```python
from build123d import *

# Parameters (mm, degrees)
ESQUISSE1_W             = 40
ESQUISSE1_H             = 35
BOSS_EXTRU_1_DEPTH      = 4
ESQUISSE2_R             = 10
ENL_V_MAT_EXTRU_1_DEPTH = 2
ENL_V_MAT_EXTRU_2_DEPTH = 27.874709301
BOSS_EXTRU_2_DEPTH      = 100
BOSS_EXTRU_2_DEPTH_BACK = 9
ESQUISSE4_R             = 7
ESQUISSE5_R             = 6
ENL_V_MAT_EXTRU_5_DEPTH = 99
ENL_V_MAT_EXTRU_9_DEPTH = 99


with BuildPart() as part:
    # Esquisse1 → Boss.-Extru.1 (new body)
    with BuildSketch(Plane(origin=(0, 0, 0), x_dir=(0, 0, -1), z_dir=(1, 0, 0))):
        Rectangle(ESQUISSE1_W, ESQUISSE1_H)
    extrude(amount=BOSS_EXTRU_1_DEPTH)

    # Esquisse2 → Enlèv. mat.-Extru.1 (cut)
    with BuildSketch(Plane.ZY):
        Circle(ESQUISSE2_R)
    extrude(amount=-ENL_V_MAT_EXTRU_1_DEPTH, mode=Mode.SUBTRACT)

    # Esquisse3 → Enlèv. mat.-Extru.2 (cut, through all)
    with BuildSketch(Plane.ZY):
        with BuildLine():
            Line((0, -17.5), (20, -17.5))
            Line((20, -17.5), (20, 17.5))
            Line((20, 17.5), (0, 17.5))
            ThreePointArc((0, 17.5), (17.5, 0), (0, -17.5))
        make_face()
    extrude(amount=-ENL_V_MAT_EXTRU_2_DEPTH, mode=Mode.SUBTRACT)

    # Esquisse4 → Boss.-Extru.2 (add, two sides: drawn at the far end of the back side and taken through both)
    with BuildSketch(Plane(origin=(0, 0, -20), x_dir=(-1, 0, 0), z_dir=(0, 0, -1)).offset(-BOSS_EXTRU_2_DEPTH_BACK)):
        with Locations((-6, 0)):
            Circle(ESQUISSE4_R)
    extrude(amount=BOSS_EXTRU_2_DEPTH + BOSS_EXTRU_2_DEPTH_BACK)

    # Esquisse5 → Enlèv. mat.-Extru.5 (cut)
    with BuildSketch(Plane(origin=(0, 0, -120), x_dir=(-1, 0, 0), z_dir=(0, 0, -1))):
        with Locations((-6, 0)):
            Circle(ESQUISSE5_R)
    extrude(amount=-ENL_V_MAT_EXTRU_5_DEPTH, mode=Mode.SUBTRACT)

    # Esquisse10 → Enlèv. mat.-Extru.9 (cut)
    with BuildSketch(Plane.XY.offset(-11)):
        with BuildLine():
            Line((6, -4), (6, 4))
            ThreePointArc((6, 4), (10, 0), (6, -4))
        make_face()
    extrude(amount=-ENL_V_MAT_EXTRU_9_DEPTH, mode=Mode.SUBTRACT)


solid = part.part
```
Read the model definition and answer for the solid it produces. Units are mm, in the model's axes. A direction names the side the tool comes from. Give positions to 0.01 mm unless a question says otherwise; leave off trailing zeros. Order: outer loops, then holes, each group sorted by start corner. A loop starts at its lowest first (then second) coordinate and runs counter-clockwise, first axis right, second up.
(1) Straight lines are drawn through the part: L1, parallel to Y at x = 6, z = -72.5; L2, parallel to X at y = -5, z = -96; L3, parallel to X at y = -2.5, z = -35.5. For each, find the intervals that lie inside material, in ascending order.
(2) For a pull along X with two mould halves and no side action, classify faces 6 (the flat face through (2, 0, 0)), 7 (the flat face through (5, 0, -21)), 8 (the cylindrical face through (1.972, 0.385, 17.496)) as released by +X, released by -X, zero draft, split by the parting line, or undercut.
(3) Find section D-D (y = -8.5). Give the vertices of the cut face in (x, z).
(4) Find section B-B (x = 7.5). Give the vertices of the cut face in (y, z).
(5) Find section C-C (z = -37.5). Give the vertices of the cut face in (x, y).
(6) Find section A-A (y = 0). Give the vertices of the cut face in (x, z).
(7) For faces 1 (the cylindrical face through (0.99, -9.76, -2.17)), 2 (the flat face through (5.6, 0.1, -11)), 3 (the flat face through (2, -17.5, -10)), 4 (the flat face through (6, 0, -16)), 5 (the cylindrical face through (13, 0, -65)), determine the directions among +Z, -Z, +X, -X, +Y, -Y from which every point of the face is accessible in a straight line to the end or side of a thin tool.
(8) Given pin 1 (1 mm diameter, centred on x = 1, y = -10.5, fed in from +Z); pin 2 (1.2 mm diameter, centred on x = 1, y = 12.5, fed in from -Z); pin 3 (2 mm diameter, centred on y = 6, z = -63.5, fed in from +X), each flat-ended and moving along its own axis, determine where each tip first touches the part or whether it passes through.
Result sheet:
1. L1: y = -7 to -6, 6 to 7
1. L2: x = 1.1 to 2.68, 9.32 to 10.9
1. L3: x = -0.54 to 0.55, 11.45 to 12.54
2. face 6: released by -X
2. face 7: undercut
2. face 8: zero draft
3. outline: (0, -20) - (4, -20) - (4, 15.3) - (0, 15.3) - (0, 5.27) - (2, 5.27) - (2, -5.27) - (0, -5.27) - close
4. outline: (-6.84, -120) - (-5.81, -120) - (-5.81, -21) - (-3.71, -21) - (-3.71, -11) - (-6.84, -11) - close; (3.71, -21) - (5.81, -21) - (5.81, -120) - (6.84, -120) - (6.84, -11) - (3.71, -11) - close
5. outline: circle Ø14 at (6, 0); hole circle Ø12 at (6, 0)
6. outline: (-1, -120) - (0, -120) - (0, -21) - (6, -21) - (6, -11) - (4, -11) - (4, 17.5) - (0, 17.5) - (0, 10) - (2, 10) - (2, -10) - (0, -10) - (0, -11) - (-1, -11) - close; (10, -21) - (12, -21) - (12, -120) - (13, -120) - (13, -11) - (10, -11) - close
7. face 1: -X
7. face 2: +Z, +X, +Y, -Y
7. face 3: +Z, -Z, +X, -X, -Y
7. face 4: +Z, -Z
7. face 5: -Z
8. pin 1: stops at z = 14.36
8. pin 2: stops at z = -20
8. pin 3: stops at x = 10.9
